Geometry: final body of the model. Coordinates: model frame, mm. A direction names the side the tool comes from. Coordinates: 2 decimals unless noted, no trailing zeros. Order: outer loops, then holes, each group sorted by start corner. A loop starts at its lowest first (then second) coordinate and runs counter-clockwise, first axis right, second up. Notation, with made-up numbers: M 69,79.5 L 110,79.5 A19 ccw 110,96.5 Z; hole C 32.5,80.5 d5. An arc over 180 degrees is marked long. Write item = value, one per line.
Autodesk Inventor part; units mm, degrees
ref_plane "YZ Plane" through (0, 0, 0) normal (1, 0, 0) x (0, 1, 0)
ref_plane "XZ Plane" through (0, 0, 0) normal (0, 1, 0) x (-1, 0, 0)
ref_plane "XY Plane" through (0, 0, 0) normal (0, 0, 1) x (1, 0, 0)
sketch "Sketch1" plane through (0, 0, 0) normal (0, 0, 1) x (1, 0, 0)
  line L0 (0, 0) -> (304.8, 0) construction
  line L1 (304.8, 0) -> (304.8, 50.8) construction
  line L2 (304.8, 50.8) -> (0, 50.8) construction
  line L3 (0, 50.8) -> (0, 0) construction
  circle A0 centre (152.4, 25.4) radius 17.4625
  circle A1 centre (152.4, 25.4) radius 30.48 construction
  circle A2 centre (152.4, 25.4) radius 22.225 construction
  line L4 (152.4, 25.4) -> (138.5082, 62.9697) construction
  circle A3 centre (138.5082, 62.9697) radius 9.525 construction
  circle A4 centre (138.5082, 62.9697) radius 17.78 construction
  circle A5 centre (89.9711, 85.09) radius 31.75 construction
  circle A6 centre (160.9785, 111.3458) radius 31.75 construction
  circle A7 centre (221.9701, 85.09) radius 31.75 construction
  line L5 (0, 50.8) -> (0, 53.34) construction
  line L6 (0, 53.34) -> (304.8, 53.34) construction
  line L7 (304.8, 53.34) -> (304.8, 50.8) construction
  circle A8 centre (138.5082, 62.9697) radius 21.59 construction
  circle A9 centre (152.4, 25.4) radius 46.99 construction
  circle A10 centre (152.4, 25.4) radius 50.8 construction
  arc A11 (84.9408, 79.3264) -> (90.9184, 92.6811) centre (89.9711, 85.09) ccw construction
  circle A12 centre (160.9785, 111.3458) radius 7.65 construction
  arc A13 (221.6946, 92.735) -> (225.5172, 78.312) centre (221.9701, 85.09) ccw construction
  circle A14 centre (160.9785, 111.3458) radius 9.1
  circle A15 centre (138.5082, 62.9697) radius 22.9 construction
  line L8 (84.9408, 79.3264) -> (123.4503, 45.7166) construction
  line L9 (168.5483, 110.2412) -> (161.1682, 59.6633) construction
  line L10 (90.9184, 92.6811) -> (89.9711, 85.09) construction
  line L11 (89.9711, 85.09) -> (84.9408, 79.3264) construction
  circle A16 centre (126.192, 96.2783) radius 3.175
  circle A17 centre (126.192, 96.2783) radius 7.9375 construction
  line L12 (90.9184, 92.6811) -> (125.2091, 88.4019) construction
  line L13 (132.0626, 90.936) -> (155.3205, 116.4945) construction
  line L14 (155.3205, 116.4945) -> (160.9785, 111.3458) construction
  line L15 (168.5483, 110.2412) -> (160.9785, 111.3458) construction
  line L16 (138.5082, 62.9697) -> (126.192, 96.2783) construction
  line L17 (89.9711, 85.09) -> (160.9785, 111.3458) construction
  line L18 (152.4, 25.4) -> (89.9711, 85.09) construction
  line L19 (152.4, 25.4) -> (160.9785, 111.3458) construction
  circle A18 centre (126.192, 96.2783) radius 9.2075 construction
  circle A19 centre (126.192, 96.2783) radius 6.1595 construction
  arc A20 (90.9184, 92.6811) -> (84.9408, 79.3264) centre (89.9711, 85.09) ccw construction
  circle A21 centre (160.9785, 111.3458) radius 25.4 construction
  circle A22 centre (221.9701, 85.09) radius 25.4 construction
  line L20 (102.9424, 114.0695) -> (76.9998, 56.1105) construction
  circle A23 centre (89.9711, 85.09) radius 25.4 construction
  line L21 (213.8361, 115.7804) -> (230.1041, 54.3996) construction
  line L22 (54.4111, 146.9058) -> (257.6111, 146.9058)
  line L23 (257.6111, 146.9058) -> (257.6111, -11.8442)
  line L24 (257.6111, -11.8442) -> (54.4111, -11.8442)
  line L25 (54.4111, -11.8442) -> (54.4111, 146.9058)
  circle A24 centre (138.5082, 62.9697) radius 14.2875
  arc A25 (225.3129, 75.4455) -> (221.0936, 95.3227) centre (223.2033, 85.3841) ccw
  line L26 (220.7531, 84.7347) -> (228.4773, 60.5377) construction
  line L27 (223.2033, 85.3841) -> (228.4773, 60.5377) construction
  line L28 (220.7531, 84.7347) -> (213.029, 108.9318) construction
  line L29 (223.2033, 85.3841) -> (217.9292, 110.2305) construction
  arc A26 (212.3049, 111.2003) -> (213.7531, 106.6633) centre (213.029, 108.9318) ccw
  arc A27 (218.4237, 107.9012) -> (217.4348, 112.5599) centre (217.9292, 110.2305) ccw
  arc A28 (218.4237, 107.9012) -> (213.7531, 106.6633) centre (228.4773, 60.5377) ccw
  arc A29 (217.4348, 112.5599) -> (212.3049, 111.2003) centre (228.4773, 60.5377) ccw
  line L30 (213.029, 108.9318) -> (212.3049, 111.2003) construction
  line L31 (217.9292, 110.2305) -> (217.4348, 112.5599) construction
  arc A30 (221.0936, 95.3227) -> (217.6635, 94.4136) centre (228.4773, 60.5377) ccw
  arc A31 (225.3129, 75.4455) -> (223.8428, 75.0559) centre (228.4773, 60.5377) ccw
  line L32 (102.6358, 107.1803) -> (91.1149, 84.5434) construction
  line L33 (79.5941, 61.9064) -> (88.8014, 85.5789) construction
  arc A32 (98.8719, 111.4706) -> (97.1455, 107.0321) centre (98.0087, 109.2513) ccw
  arc A33 (101.5557, 105.0581) -> (103.7158, 109.3025) centre (102.6358, 107.1803) ccw
  arc A34 (101.5557, 105.0581) -> (97.1455, 107.0321) centre (79.5941, 61.9064) ccw
  line L34 (98.0087, 109.2513) -> (98.8719, 111.4706) construction
  line L35 (102.6358, 107.1803) -> (103.7158, 109.3025) construction
  arc A35 (103.7158, 109.3025) -> (98.8719, 111.4706) centre (79.5941, 61.9064) ccw
  arc A36 (217.6635, 94.4136) -> (223.8428, 75.0559) centre (220.7531, 84.7347) ccw
  arc A37 (86.5066, 75.4886) -> (95.7233, 93.5981) centre (91.1149, 84.5434) ccw
  line L36 (88.8014, 85.5789) -> (98.0087, 109.2513) construction
  line L37 (91.1149, 84.5434) -> (79.5941, 61.9064) construction
  arc A38 (86.5066, 75.4886) -> (85.1185, 76.1099) centre (79.5941, 61.9064) ccw
  arc A39 (95.7233, 93.5981) -> (92.4843, 95.0479) centre (79.5941, 61.9064) ccw
  arc A40 (92.4843, 95.0479) -> (85.1185, 76.1099) centre (88.8014, 85.5789) ccw
  line L38 (160.9785, 111.3458) -> (138.0151, 122.2014) construction
  line L39 (160.9785, 111.3458) -> (183.9418, 100.4902) construction
  circle A41 centre (138.5082, 62.9697) radius 26.75 construction
  line L40 (221.6946, 92.735) -> (137.5448, 89.7024) construction
  line L41 (225.5172, 78.312) -> (150.9113, 39.269) construction
  line L42 (221.9701, 85.09) -> (221.6946, 92.735) construction
  line L43 (221.9701, 85.09) -> (225.5172, 78.312) construction
  line L44 (138.5082, 62.9697) -> (137.5448, 89.7024) construction
  line L45 (138.5082, 62.9697) -> (150.9113, 39.269) construction
  arc A42 (225.5172, 78.312) -> (221.6946, 92.735) centre (221.9701, 85.09) ccw construction
  arc A43 (225.5172, 78.312) -> (224.7763, 77.9733) centre (221.9701, 85.09) ccw construction
  line L46 (138.5082, 62.9697) -> (221.9701, 85.09) construction
  line L47 (152.4, 25.4) -> (176.2235, 34.209) construction
  line L48 (152.4, 25.4) -> (128.5765, 16.591) construction
  point P0 (215.4629, 109.6423)
  point P1 (100.3481, 108.2736)
  dimension "d1" = 50.8
  dimension "d2" = 34.925
  dimension "d3" = 25.4
  dimension "d4" = 152.4
  dimension "d7" = 60.96
  dimension "d8" = 44.45
  dimension "d9" = 19.05
  dimension "d10" = 35.56
  dimension "d11" = 40.0558
  dimension "d12" = 63.5
  dimension "d13" = 63.5
  dimension "d14" = 63.5
  dimension "d15" = 2.54
  dimension "d16" = 304.8
  dimension "d17" = 43.18
  dimension "d18" = 93.98
  dimension "d19" = 101.6
  dimension "d21" = 15.3
  dimension "d22" = 15.3
  dimension "d24" = 18.2
  dimension "d29" = 45.8
  dimension "d30" = 146
  dimension "d31" = 6.35
  dimension "d32" = 15.875
  dimension "d33" = 146
  dimension "d35" = 18.415
  dimension "d37" = 12.319
  dimension "d40" = 50.8
  dimension "d41" = 50.8
  dimension "d42" = 17
  dimension "d43" = 17
  dimension "d44" = 50.8
  dimension "d53" = 203.2
  dimension "d54" = 158.75
  dimension "d55" = 35.56
  dimension "d56" = 35.56
  dimension "d57" = 28.575
  dimension "d67" = 25.4
  dimension "d68" = 25.4
  dimension "d69" = 2.86
  dimension "d70" = 25.4
  dimension "d71" = 25.4
  dimension "d72" = 4.7625
  dimension "d75" = 2.86
  dimension "d80" = 4.7625
  dimension "d82" = 4.7625
  dimension "d83" = 50.8
  dimension "d84" = 50.8
  dimension "d85" = 10.16
  dimension "d97" = 48.4188
  dimension "d99" = 20.32
  dimension "d101" = 25.4
  dimension "d102" = 25.4
  dimension "d103" = 10.16
  dimension "d105" = 17
  dimension "d106" = 17
  dimension "d107" = 53.5
  dimension "d108" = 154.44
  dimension "d109" = 7.65
  dimension "d111" = 86.3435
  dimension "d112" = 12.78
  dimension "d113" = 12.78
  dimension "d123" = 25.4
  dimension "d124" = 25.4
extrude "Extrusion3" add sketch "Sketch1" against normal blind 6.35
hole "Hole3" at (79.5941, 61.9064, 0) at (228.4773, 60.5377, 0) at (183.9418, 100.4902, 0) at (138.0151, 122.2014, 0) direction (0, 0, -1) diameter 4.7625 end through all
hole "Hole4" at (128.5765, 16.591, 0) at (176.2235, 34.209, 0) direction (0, 0, -1) diameter 3.9624 end through all
equation "\"d7\" = Gear48tPD"
equation "\"d8\" = Gear35tPD"
equation "\"d9\" = Gear15tPD"
equation "\"d10\" = Gear28tPD"
equation "\"d11\" = 0.5 * Gear48tPD + 0.5 * Gear15tPD + MeshingClearance"
equation "\"d12\" = CimOD"
equation "\"d13\" = CimOD"
equation "\"d14\" = CimOD"
equation "\"d17\" = Gear28tPD + ClearanceDiameter"
equation "\"d18\" = WheelOD"
equation "\"d19\" = WheelClearance"
equation "\"Pulley48tPD\" = 45.8"
equation "\"Pulley19tPD\" = 18.2"
equation "\"Pulley16tPD\" = 15.3"
equation "\"Gear15tPD\" = 19.05"
equation "\"Gear35tPD\" = 44.45"
equation "\"Gear48tPD\" = 60.96"
equation "\"Gear28tPD\" = 35.56"
equation "\"BearingLargeOD\" = 28.575"
equation "\"BearingSmallOD\" = 22.225"
equation "\"MeshingClearance\" = 0.0508"
equation "\"CimOD\" = 63.5"
equation "\"WheelOD\" = 93.98"
equation "\"ClearanceDiameter\" = 7.62"
equation "\"WheelClearance\" = 101.6"
equation "\"TensioningBearingID\" = 6.35"
equation "\"TensioningBearingOD\" = 15.875"
equation "\"SpingClipClearance\" = 8.89"
equation "\"Pi\" = 79.79645"
equation "\"Pulley56tPD\" = 53.5"
equation "\"BearingXLargeOD\" = 34.925"
properties part number "OutlineSketch1" material "Aluminum 6061"
1) Mould query, pull axis X, two halves, no side actions, for faces 1 (the face through (95.809, 110.163, -3.131)), 2 (the face through (155, 69, -6.35)). Classes: pulls with the +X half, pulls with the -X half, needs draft (parallel to the pull), parting line crosses it, or undercut.
Numbers:
face_1 = undercut
face_2 = needs draft
2) Set-up query: faces 3 (the face through (216.11, 107.35, -3.13)), 4 (the face through (155, 146.906, -3)). Return all of +Z, -Z, +X, -X, +Y, -Y with unobstructed straight access to the full face (end or side cutting, diameter ignored); none if empty.
Numbers:
face_3 = +Z, -Z
face_4 = +Z, -Z, +X, -X, +Y
3) Line query: L1, parallel to X at y = 25, z = -3.25; L2, parallel to Y at x = 162.5, z = -0.5; L3, parallel to Y at x = 176, z = -5. Output: solid intervals per line, ascending.
Numbers:
L1 = 54.41 to 134.94, 169.86 to 257.61
L2 = -11.84 to 11.15, 39.65 to 102.37, 120.32 to 146.91
L3 = -11.84 to 32.24, 36.18 to 146.91
4) Section C-C, the plane y = 82. Return loops of the section in (x, z), and give its area (3 significant figures).
Numbers:
outline = M 54.41,-6.35 L 79.29,-6.35 L 79.29,0 L 54.41,0 Z; M 100.95,-6.35 L 210.97,-6.35 L 210.97,0 L 100.95,0 Z; M 232.78,-6.35 L 257.61,-6.35 L 257.61,0 L 232.78,0 Z
area = 1,010 mm²
5) Pin query (flat end, axial travel): pin 1 (11 mm diameter, centred on x = 160.98, y = 111.35, fed in from -Z). Return the tip coordinate at first contact, or that it passes through.
Numbers:
pin_1 = through
6) Section A-A, the plane y = 25.4. Return loops of the section in (x, z), and give its area (3 significant figures).
Numbers:
outline = M 54.41,-6.35 L 134.94,-6.35 L 134.94,0 L 54.41,0 Z; M 169.86,-6.35 L 257.61,-6.35 L 257.61,0 L 169.86,0 Z
area = 1,070 mm²
7) Section B-B, the plane z = -3.25. Give the number of separate pieces and of enclosed holes in the cut face, and give its area (3 significant figures).
Numbers:
separate_pieces = 1
enclosed_holes = 14
area = 29,400 mm²
